```python
from build123d import *

# Parameters (mm, degrees)
CROQUIS1_W              = 162.4
CROQUIS1_H              = 6.2
CROQUIS1_R              = 1.5
SALIENTE_EXTRUIR1_DEPTH = 6.2
CROQUIS2_R              = 1.5
CORTAR_EXTRUIR1_DEPTH   = 6.2


with BuildPart() as part:
    # Croquis1 → Saliente-Extruir1 (new body)
    with BuildSketch(Plane.XY):
        Rectangle(CROQUIS1_W, CROQUIS1_H)
        with Locations((-71.5, 0)):
            Circle(CROQUIS1_R, mode=Mode.SUBTRACT)
        Circle(CROQUIS1_R, mode=Mode.SUBTRACT)
        with Locations((71.5, 0)):
            Circle(CROQUIS1_R, mode=Mode.SUBTRACT)
    extrude(amount=SALIENTE_EXTRUIR1_DEPTH)

    # Croquis2 → Cortar-Extruir1 (cut)
    with BuildSketch(Plane(origin=(0, 3.1, 0), x_dir=(1, 0, 0), z_dir=(0, 1, 0))):
        with Locations((-77.5, -3.1)):
            Circle(CROQUIS2_R)
        with Locations((-28.5, -3.1)):
            Circle(CROQUIS2_R)
        with Locations((28.5, -3.1)):
            Circle(CROQUIS2_R)
        with Locations((77.5, -3.1)):
            Circle(CROQUIS2_R)
    extrude(amount=-CORTAR_EXTRUIR1_DEPTH, mode=Mode.SUBTRACT)


solid = part.part
```
Input: part model. Units: mm. Frame: model coordinates. Give positions to 0.01 mm unless a question says otherwise; leave off trailing zeros. Write each loop counter-clockwise with the first axis right and the second up, starting at its lowest first coordinate (ties: lowest second). Pieces come first, ordered by that corner, then holes. Notation, with made-up numbers: (42, 14) - (76, 14) arc R25 cw to (76, 48) - close; hole circle Ø6 at (62.25, -24). An arc over 180 degrees is marked (long way). Write item = value, one per line. Start each with the question number.
1. Section query B-B, the plane x = -77.5. Output: boundary loops of the cut face in (y, z).
2. Mould query, pull axis X, two halves, no side actions, for faces 1 (the flat face through (-81.2, 0, 3)), 2 (the flat face through (81.2, 0, 3)), 3 (the cylindrical face through (73, 0, 3)), 4 (the flat face through (-1.1, 1.4, 6.2)). Classes: released by +X, released by -X, zero draft, split by the parting line, or undercut.
3. Section query A-A, the plane y = 0. Output: boundary loops of the cut face in (x, z), then the cut area to 3 significant figures.
4. Ray query, L1, parallel to X at y = 1.75, z = 3.25; L2, parallel to Z at x = 28.5, y = 0.25; L3, parallel to Y at x = -71.5, z = 5.25. Return the intervals inside material, ascending.
5. First-contact query: pin 1 Ø2.5 at (x, z) = (77.5, 3.1) entering from +Y; pin 2 Ø3.5 at (x, z) = (-28.5, 3.1) entering from -Y. Flat tips, straight axial feed; report the tip coordinate or a pass-through.
Check sheet entries:
q1.outline = (-3.1, 0) - (3.1, 0) - (3.1, 1.6) - (-3.1, 1.6) - close; (-3.1, 4.6) - (3.1, 4.6) - (3.1, 6.2) - (-3.1, 6.2) - close
q2.face_1 = released by -X
q2.face_2 = released by +X
q2.face_3 = undercut
q2.face_4 = zero draft
q3.outline = (-81.2, 0) - (-73, 0) - (-73, 6.2) - (-81.2, 6.2) - close; (-70, 0) - (-1.5, 0) - (-1.5, 6.2) - (-70, 6.2) - close; (1.5, 0) - (70, 0) - (70, 6.2) - (1.5, 6.2) - close; (73, 0) - (81.2, 0) - (81.2, 6.2) - (73, 6.2) - close; hole circle Ø3 at (-77.5, 3.1); hole circle Ø3 at (-28.5, 3.1); hole circle Ø3 at (28.5, 3.1); hole circle Ø3 at (77.5, 3.1)
q3.area = 923 mm2
q4.L1 = -81.2 to -78.99, -76.01 to -29.99, -27.01 to 27.01, 29.99 to 76.01, 78.99 to 81.2
q4.L2 = 0 to 1.6, 4.6 to 6.2
q4.L3 = -3.1 to -1.5, 1.5 to 3.1
q5.pin_1 = through
q5.pin_2 = -3.1
